```python
from build123d import *

# Parameters (mm, degrees)
EXTRUDE_1_DEPTH     = 120
FILLET_1_R          = 0.5
CUT_EXTRUDE_1_DEPTH = 48
SKETCH_5_R          = 2.0500000000000123
SKETCH_5_R_2        = 2.0500000000000056
SKETCH_5_R_3        = 2.0499999999999923
CUT_EXTRUDE_2_DEPTH = 5
SKETCH_6_R          = 70.99685128536404
CUT_EXTRUDE_3_DEPTH = 185.82965146426048


with BuildPart() as part:
    # 草图3 → 凸台-拉伸1 (new, symmetric)
    with BuildSketch(Plane.XY):
        with BuildLine():
            Line((131, -50.99999999999999), (6.25e-15, -51))
            ThreePointArc((6.25e-15, -51), (36.062445840513924, -36.062445840513924), (51, 0))
            ThreePointArc((51, 0), (89.3844868048509, -28.034138345331712), (131, -50.99999999999999))
        make_face()
    extrude(amount=EXTRUDE_1_DEPTH, both=True)

    # 圆角1
    fillet_1_edges = [part.edges().sort_by_distance(p)[0] for p in [
        (50.99999999999999, -2.664e-14, 0),
        (6.25e-15, -51, 0),
    ]]
    fillet(fillet_1_edges, radius=FILLET_1_R)

    # 草图4 → 切除-拉伸1 (cut)
    with BuildSketch(Plane(origin=(0, 0, 0), x_dir=(1, 0, 0), z_dir=(0, 1, 0))):
        Polygon((124.4641016151378, -112), (124.4641016151378, -108), (121.00000000000006, -106.00000000000001), (117.5358983848623, -108), (117.5358983848623, -112), (121.00000000000004, -113.99999999999999), align=None)
        Polygon((29.599504938362088, -106.00000000000001), (26.135403323224345, -108.00000000000001), (26.135403323224345, -112), (29.599504938362088, -113.99999999999999), (33.06360655349983, -112), (33.06360655349983, -108.00000000000001), align=None)
        Polygon((33.06360655349983, 108.00000000000001), (29.599504938362088, 106.00000000000001), (26.135403323224345, 108.00000000000001), (26.135403323224345, 112), (29.599504938362088, 113.99999999999999), (33.06360655349983, 112), align=None)
        Polygon((121.00000000000004, 113.99999999999999), (124.4641016151378, 112), (124.4641016151378, 108), (121.00000000000006, 106.00000000000001), (117.5358983848623, 108), (117.5358983848623, 112), align=None)
        Polygon((123.00000000000004, -36.53589838486225), (119.00000000000006, -36.53589838486225), (117.00000000000004, -39.99999999999999), (119.00000000000004, -43.46410161513774), (123.00000000000003, -43.46410161513774), (125.00000000000006, -39.99999999999999), align=None)
        Polygon((125.00000000000003, 40.00000000000008), (123.00000000000001, 43.464101615137785), (119.00000000000001, 43.464101615137785), (116.99999999999999, 40), (118.99999999999997, 36.535898384862286), (123.00000000000006, 36.535898384862286), align=None)
    extrude(amount=-CUT_EXTRUDE_1_DEPTH, mode=Mode.SUBTRACT)

    # 草图5 → 切除-拉伸2 (cut)
    with BuildSketch(Plane(origin=(2.54e-15, -47.99999999999999, 0), x_dir=(1, 5e-17, 0), z_dir=(-5e-17, 1, 0))):
        with Locations(Location((29.599504938362074, -110.00000000000001, 0), (0, 0, 180))):
            Circle(SKETCH_5_R)
        with Locations((29.599504938362074, 110.00000000000001)):
            Circle(SKETCH_5_R)
        with Locations(Location((121, 110.00000000000001, 0), (0, 0, 180))):
            Circle(SKETCH_5_R_2)
        with Locations((121.00000000000006, -110)):
            Circle(SKETCH_5_R_2)
        with Locations(Location((120.94806034143625, 40.089962127560234, 0), (0, 0, 180))):
            Circle(SKETCH_5_R_3)
        with Locations(Location((121.00000000000006, -40, 0), (0, 0, 180))):
            Circle(SKETCH_5_R_3)
    extrude(amount=-CUT_EXTRUDE_2_DEPTH, mode=Mode.SUBTRACT)

    # 草图6 → 切除-拉伸3 (cut, through all)
    with BuildSketch(Plane.XY):
        with Locations((70.54975246918104, -50.99999999999999)):
            Circle(SKETCH_6_R)
    extrude(amount=CUT_EXTRUDE_3_DEPTH, mode=Mode.SUBTRACT)


solid = part.part
```
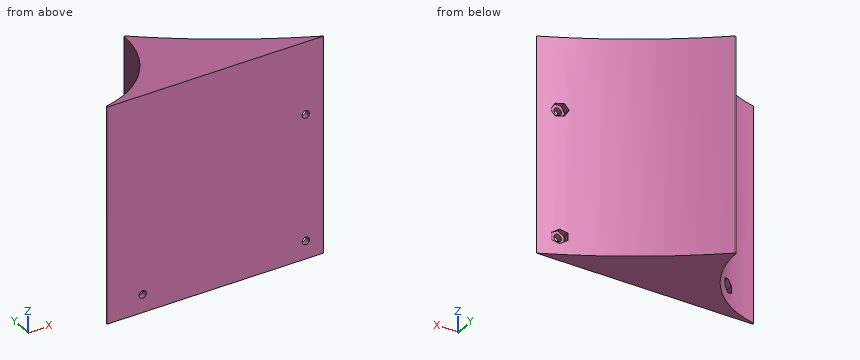
The listing builds one solid part. Answer for the finished solid, in the listing's coordinates (mm). Give positions to 0.01 mm unless a question says otherwise; leave off trailing zeros. Order: outer loops, then holes, each group sorted by start corner. A loop starts at its lowest first (then second) coordinate and runs counter-clockwise, first axis right, second up. Notation, with made-up numbers: (86, 70) -> (121, 70) arc R16 ccw to (121, 101) -> close; hole circle Ø7 at (20.5, -21.75). An arc over 180 degrees is marked (long way). Answer as a JSON object with one key per item and string values. Group by question number.
Item 1: The part is cut by section B-B on y = -35. Write down the section's boundary in (x, z).
Item 2: The part is cut by section C-C on x = 63. Write down the section's boundary in (y, z), and give its area (3 significant figures).
Item 3: The part is cut by section A-A on z = -110. Give the number of separate pieces and of enclosed holes in the cut face, and give its area (3 significant figures).
Item 4: Flat-ended cylindrical pins translate along their axes: pin 1 (2 mm diameter, centred on y = -46.5, z = -110.5, fed in from +X); pin 2 (8 mm diameter, centred on y = -23, z = -61, fed in from +X); pin 3 (7.5 mm diameter, centred on x = 122.5, z = -39.5, fed in from +Y). Find the tip coordinate at first contact, or state that the pin passes through.
Item 5: Consider L1, parallel to Z at x = 121, y = -48.7; L2, parallel to Y at x = 26, z = -100; L3, parallel to Y at x = 28, z = -62. Determine where each line is inside the solid, lowest interval first. Write a range as from..to.
Result set:
{
 "1": {"outline": "(37.09, -120) -> (100.75, -120) -> (100.75, 0) -> (37.09, 0) -> close"},
 "2": {"outline": "(-51, -120) -> (-9.58, -120) -> (-9.58, 0) -> (-51, 0) -> close", "area": "4,970 mm²"},
 "3": {"separate pieces": "3", "enclosed holes": "0", "area": "2,320 mm²"},
 "4": {"pin 1": "x = 117.54", "pin 2": "x = 87.77", "pin 3": "y = -45.69"},
 "5": {"L1": "-120..-112.05, -107.95..-42.14, -38.04..0", "L2": "-51..-43.87", "L3": "-51..-42.63"}
}
